For this review, take the finished solid that the model builds, in its own axes (mm). Face numbers are marked on the shaded views. A direction names the side the tool comes from. Give positions to 0.01 mm unless a question says otherwise; leave off trailing zeros. Order: outer loops, then holes, each group sorted by start corner. A loop starts at its lowest first (then second) coordinate and runs counter-clockwise, first axis right, second up. Notation, with made-up numbers: (-35.5, 48.25) -> (5.5, 48.25) arc R11 cw to (5.5, 53.25) -> close; hole circle Ø2 at (50.25, -18.5). An arc over 180 degrees is marked (long way). Return JSON: item names as keys, results as strings. Group by question number.
1) The part is to be moulded in two halves that separate along X. For the marked faces 1 and 2, say which applies: released by +X, released by -X, zero draft, split by the parting line, or undercut.
2) Add section C-C (x = -47). Give the boundary of the cut face in (y, z) (3 decimals).
3) Add section A-A (x = -303). Give the boundary of the cut face in (y, z), then the cut area to 3 significant figures.
4) Add section B-B (y = -8). Give the boundary of the cut face in (x, z) (1 decimal), then the cut area to 3 significant figures.
5) Insertion check: P1, Ø8, axis at x = -42.5, y = -44.5, coming from the +Z side (3 decimals); P2, Ø2, axis at x = -161.5, y = 67.5, coming from the +Z side. Each pin has a flat end and moves straight along its axis. Give the tip position at first contact, or say it passes through.
6) To check wall thickness, follow line 1 along Y through (x, z) = (75, -0.5); line 2 along X through (y, z) = (28, -2); line 3 along Y through (x, z) = (-398, -2.5). State the ranges of each line that lie inside material, in increasing order.
7) For the marked faces 3 and 4, list the 3-axis set-ups (+Z, -Z, +X, -X, +Y, -Y) from which the entire face can be reached by the end or side of a thin tool; tool diameter is ignored.
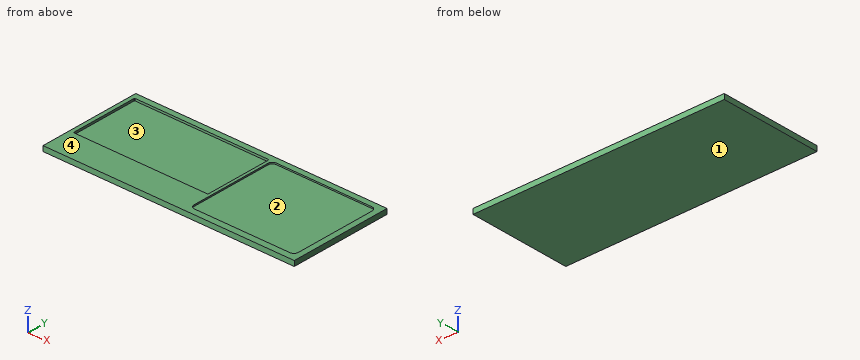
from build123d import *

# Parameters (mm, degrees)
F0_W     = 558.8
F0_H     = 228.6
F1_DEPTH = 11.43
F2_DEPTH = 4.7625
F3_DEPTH = 3.175


with BuildPart() as f1:
    # F0 (on Top) → F1 (new body)
    with BuildSketch(Plane.XY):
        with Locations((-150.8125, -0.79375)):
            Rectangle(F0_W, F0_H)
        with BuildLine():
            ThreePointArc((-421.48125, 99.21875), (-421.016282, 100.341282), (-419.89375, 100.80625))
            Line((-419.89375, 100.80625), (-123.825, 100.80625))
            ThreePointArc((-123.825, 100.80625), (-122.702468, 100.341282), (-122.2375, 99.21875))
            Line((-122.2375, 99.21875), (-122.2375, -48.41875))
            ThreePointArc((-122.2375, -48.41875), (-122.702468, -49.541282), (-123.825, -50.00625))
            Line((-123.825, -50.00625), (-419.89375, -50.00625))
            ThreePointArc((-419.89375, -50.00625), (-421.016282, -49.541282), (-421.48125, -48.41875))
            Line((-421.48125, -48.41875), (-421.48125, 99.21875))
        make_face(mode=Mode.SUBTRACT)
        with BuildLine():
            Line((-106.3625, 100.80625), (106.3625, 100.80625))
            ThreePointArc((106.3625, 100.80625), (113.097692, 98.016442), (115.8875, 91.28125))
            Line((115.8875, 91.28125), (115.8875, -91.28125))
            ThreePointArc((115.8875, -91.28125), (113.097692, -98.016442), (106.3625, -100.80625))
            Line((106.3625, -100.80625), (-106.3625, -100.80625))
            ThreePointArc((-106.3625, -100.80625), (-113.097692, -98.016442), (-115.8875, -91.28125))
            Line((-115.8875, -91.28125), (-115.8875, 91.28125))
            ThreePointArc((-115.8875, 91.28125), (-113.097692, 98.016442), (-106.3625, 100.80625))
        make_face(mode=Mode.SUBTRACT)
        with BuildLine():
            Line((-123.825, 100.80625), (-419.89375, 100.80625))
            ThreePointArc((-419.89375, 100.80625), (-421.016282, 100.341282), (-421.48125, 99.21875))
            Line((-421.48125, 99.21875), (-421.48125, -48.41875))
            ThreePointArc((-421.48125, -48.41875), (-421.016282, -49.541282), (-419.89375, -50.00625))
            Line((-419.89375, -50.00625), (-123.825, -50.00625))
            ThreePointArc((-123.825, -50.00625), (-122.702468, -49.541282), (-122.2375, -48.41875))
            Line((-122.2375, -48.41875), (-122.2375, 99.21875))
            ThreePointArc((-122.2375, 99.21875), (-122.702468, 100.341282), (-123.825, 100.80625))
        make_face()
        with BuildLine():
            ThreePointArc((115.8875, 91.28125), (113.097692, 98.016442), (106.3625, 100.80625))
            Line((106.3625, 100.80625), (-106.3625, 100.80625))
            ThreePointArc((-106.3625, 100.80625), (-113.097692, 98.016442), (-115.8875, 91.28125))
            Line((-115.8875, 91.28125), (-115.8875, -91.28125))
            ThreePointArc((-115.8875, -91.28125), (-113.097692, -98.016442), (-106.3625, -100.80625))
            Line((-106.3625, -100.80625), (106.3625, -100.80625))
            ThreePointArc((106.3625, -100.80625), (113.097692, -98.016442), (115.8875, -91.28125))
            Line((115.8875, -91.28125), (115.8875, 91.28125))
        make_face()
    extrude(amount=-F1_DEPTH)

    # F0 (on Top) → F2 (cut)
    with BuildSketch(Plane.XY):
        with BuildLine():
            Line((-123.825, 100.80625), (-419.89375, 100.80625))
            ThreePointArc((-419.89375, 100.80625), (-421.016282, 100.341282), (-421.48125, 99.21875))
            Line((-421.48125, 99.21875), (-421.48125, -48.41875))
            ThreePointArc((-421.48125, -48.41875), (-421.016282, -49.541282), (-419.89375, -50.00625))
            Line((-419.89375, -50.00625), (-123.825, -50.00625))
            ThreePointArc((-123.825, -50.00625), (-122.702468, -49.541282), (-122.2375, -48.41875))
            Line((-122.2375, -48.41875), (-122.2375, 99.21875))
            ThreePointArc((-122.2375, 99.21875), (-122.702468, 100.341282), (-123.825, 100.80625))
        make_face()
    extrude(amount=-F2_DEPTH, mode=Mode.SUBTRACT)

    # F0 (on Top) → F3 (cut)
    with BuildSketch(Plane.XY):
        with BuildLine():
            ThreePointArc((115.8875, 91.28125), (113.097692, 98.016442), (106.3625, 100.80625))
            Line((106.3625, 100.80625), (-106.3625, 100.80625))
            ThreePointArc((-106.3625, 100.80625), (-113.097692, 98.016442), (-115.8875, 91.28125))
            Line((-115.8875, 91.28125), (-115.8875, -91.28125))
            ThreePointArc((-115.8875, -91.28125), (-113.097692, -98.016442), (-106.3625, -100.80625))
            Line((-106.3625, -100.80625), (106.3625, -100.80625))
            ThreePointArc((106.3625, -100.80625), (113.097692, -98.016442), (115.8875, -91.28125))
            Line((115.8875, -91.28125), (115.8875, 91.28125))
        make_face()
    extrude(amount=-F3_DEPTH, mode=Mode.SUBTRACT)


solid = f1.part
Evaluation:
{
 "1": {"face 1": "zero draft", "face 2": "undercut"},
 "2": {"outline": "(-115.094, -11.43) -> (113.506, -11.43) -> (113.506, 0) -> (100.806, 0) -> (100.806, -3.175) -> (-100.806, -3.175) -> (-100.806, 0) -> (-115.094, 0) -> close"},
 "3": {"outline": "(-115.09, -11.43) -> (113.51, -11.43) -> (113.51, 0) -> (100.81, 0) -> (100.81, -4.76) -> (-50.01, -4.76) -> (-50.01, 0) -> (-115.09, 0) -> close", "area": "1,890 mm^2"},
 "4": {"outline": "(-430.2, -11.4) -> (128.6, -11.4) -> (128.6, 0) -> (115.9, 0) -> (115.9, -3.2) -> (-115.9, -3.2) -> (-115.9, 0) -> (-122.2, 0) -> (-122.2, -4.8) -> (-421.5, -4.8) -> (-421.5, 0) -> (-430.2, 0) -> close", "area": "4,230 mm^2"},
 "5": {"P1": "z = -3.175", "P2": "z = -4.76"},
 "6": {"line 1": "-115.09 to -100.81, 100.81 to 113.51", "line 2": "-430.21 to -421.48, -122.24 to -115.89, 115.89 to 128.59", "line 3": "-115.09 to -50.01, 100.81 to 113.51"},
 "7": {"face 3": "+Z", "face 4": "+Z, +X, -X, +Y, -Y"}
}
